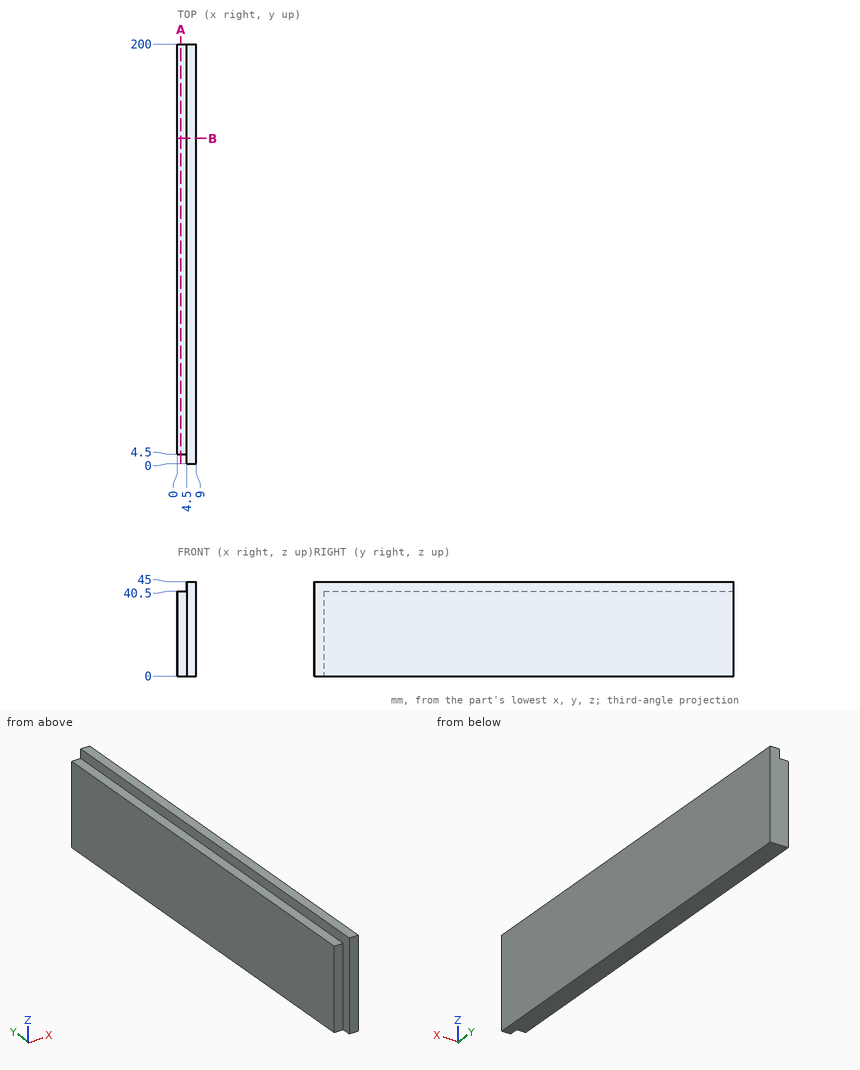
Study the drawing (mm; zero at the part's minimum x, y, z) and answer. Coordinates: 2 decimals unless noted, no trailing zeros. Loops run counter-clockwise (first coordinate to the right, second up) from the corner with the lowest first, then second, coordinate; pieces in that order, holes last. Notation, with made-up numbers: M 11,34.5 L 46,34.5 A25 ccw 46,66.5 Z; hole C -39,40 d10. An arc over 180 degrees is marked long. Answer in a Markdown table with one row per item. Add a question column.
1. Consider L1, parallel to X at y = 89.5, z = 43.5; L2, parallel to Y at x = 1.5, z = 15; L3, parallel to Z at x = 3, y = 153.5. Determine where each line is inside the solid, lowest interval first.
2. Flat-ended cylindrical pins translate along their axes: P1, Ø2, axis at x = 3, z = 25, coming from the -Y side; P2, Ø3.5, axis at x = 1.5, y = 125, coming from the +Z side. Find the tip coordinate at first contact, or state that the pin passes through.
3. Find section B-B, the plane y = 155. Write down the section's boundary in (x, z).
4. Find section A-A, the plane x = 1.75. Write down the section's boundary in (y, z), then the cut area to 3 significant figures.
Reported:
| question | item | result |
|---|---|---|
| 1 | L1 | x = 4.5 to 9 |
| 1 | L2 | y = 4.5 to 200 |
| 1 | L3 | z = 0 to 40.5 |
| 2 | P1 | stops at y = 4.5 |
| 2 | P2 | stops at z = 40.5 |
| 3 | outline | M 0,0 L 9,0 L 9,45 L 4.5,45 L 4.5,40.5 L 0,40.5 Z |
| 4 | outline | M 4.5,0 L 200,0 L 200,40.5 L 4.5,40.5 Z |
| 4 | area | 7,920 mm^2 |
